```python
from build123d import *

# Parameters (mm, degrees)
SKETCH1_W           = 82
SKETCH1_H           = 82
BOSS_EXTRUDE1_DEPTH = 2
SKETCH2_R           = 7.955
CUT_EXTRUDE1_DEPTH  = 10
CUT_EXTRUDE4_DEPTH  = 10


with BuildPart() as part:
    # Sketch1 → Boss-Extrude1 (new body)
    with BuildSketch(Plane(origin=(0, 0, 0), x_dir=(1, 0, 0), z_dir=(0, 1, 0))):
        Rectangle(SKETCH1_W, SKETCH1_H)
    extrude(amount=BOSS_EXTRUDE1_DEPTH)

    # Sketch2 → Cut-Extrude1 (cut)
    with BuildSketch(Plane(origin=(0, 2, 0), x_dir=(1, 0, 0), z_dir=(0, 1, 0))):
        with Locations(Location((-12.87, 0, 0), (0, 0, 270))):
            Circle(SKETCH2_R)
        with Locations(Location((12.87, 0, 0), (0, 0, 270))):
            Circle(SKETCH2_R)
    extrude(amount=-CUT_EXTRUDE1_DEPTH, mode=Mode.SUBTRACT)

    # Sketch6 → Cut-Extrude4 (cut)
    with BuildSketch(Plane(origin=(0, 2, 0), x_dir=(1, 0, 0), z_dir=(0, 1, 0))):
        Polygon((-1.5, 22.5), (1.5, 22.5), (1.5, 28.3), (4, 28.3), (4, 31.75), (1.5, 31.75), (1.5, 41), (-1.5, 41), (-1.5, 31.75), (-4, 31.75), (-4, 28.3), (-1.5, 28.3), align=None)
        Polygon((28.3, 1.5), (28.3, 4), (31.75, 4), (31.75, 1.5), (41, 1.5), (41, -1.5), (31.75, -1.5), (31.75, -4), (28.3, -4), (28.3, -1.5), (22.5, -1.5), (22.5, 1.5), align=None)
        Polygon((1.5, -28.3), (4, -28.3), (4, -31.75), (1.5, -31.75), (1.5, -41), (-1.5, -41), (-1.5, -31.75), (-4, -31.75), (-4, -28.3), (-1.5, -28.3), (-1.5, -22.5), (1.5, -22.5), align=None)
        Polygon((-28.3, -1.5), (-28.3, -4), (-31.75, -4), (-31.75, -1.5), (-41, -1.5), (-41, 1.5), (-31.75, 1.5), (-31.75, 4), (-28.3, 4), (-28.3, 1.5), (-22.5, 1.5), (-22.5, -1.5), align=None)
    extrude(amount=-CUT_EXTRUDE4_DEPTH, mode=Mode.SUBTRACT)


solid = part.part
```
Part model, mm, in its own coordinate system. A direction names the side the tool comes from. Give positions to 0.01 mm unless a question says otherwise; leave off trailing zeros. Order: outer loops, then holes, each group sorted by start corner. A loop starts at its lowest first (then second) coordinate and runs counter-clockwise, first axis right, second up. Notation, with made-up numbers: M 21.5,-27.75 L 59.5,-27.75 A26 ccw 59.5,8.25 Z; hole C 49.25,-11.75 d6. An arc over 180 degrees is marked long. Use a Markdown table: item, result. Add a question column.
(1) Probe line 1 along X through (y, z) = (1.45, 0) (3 decimals); line 2 along Z through (x, y) = (29, 1.5); line 3 along Z through (x, y) = (26, 0.9). List the from-to ranges inside material, lowest first. Write a range as [from, to].
(2) Mould opens along Z. For faces 1 (the face through (0, 1, 22.5)), 2 (the face through (-1.5, 1, -36)), 3 (the face through (-36, 1, 1.5)), 4 (the face through (4, 1, 30)) say: +Z half, -Z half, draft (parallel to the pull), parting line (faces both ways), or undercut.
(3) 3-axis set-ups, long thin cutter, end or side, ignore diameter. For faces 5 (the face through (-1.5, 1, 36)), 6 (the face through (-25, 1, 1.5)), 7 (the face through (-3, 1, -28.3)): which of +Z, -Z, +X, -X, +Y, -Y reach the whole face in a straight line?
(4) Drop a flat-ended pin along its axis: P1, Ø4, axis at x = 8.5, z = 2.5, coming from the +Y side. Give the stop position or say it passes through.
(5) Saw through at D-D, the plane x = 24. Give the cut face in (y, z).
(6) Saw through at C-C, the plane y = 1.3. Give the number of separate pieces and of enclosed holes in the cut face, and give its area (3 significant figures).
(7) Saw through at A-A, the plane x = 12.87. Give the cut face in (y, z) (3 decimals), and give its area (3 significant figures).
(8) Saw through at B-B, the plane z = 0. Give the cut face in (x, y) (3 decimals), and give its area (3 significant figures).
Answer key:
| question | item | result |
|---|---|---|
| 1 | line 1 | [-22.5, -20.825], [-4.915, 4.915], [20.825, 22.5] |
| 1 | line 2 | [-41, -4], [4, 41] |
| 1 | line 3 | [-41, -1.5], [1.5, 41] |
| 2 | face 1 | +Z half |
| 2 | face 2 | draft |
| 2 | face 3 | undercut |
| 2 | face 4 | undercut |
| 3 | face 5 | +Z, +Y, -Y |
| 3 | face 6 | -X, +Y, -Y |
| 3 | face 7 | +Y, -Y |
| 4 | P1 | through |
| 5 | outline | M 0,-41 L 2,-41 L 2,-1.5 L 0,-1.5 Z; M 0,1.5 L 2,1.5 L 2,41 L 0,41 Z |
| 6 | separate pieces | 1 |
| 6 | enclosed holes | 2 |
| 6 | area | 6,040 mm^2 |
| 7 | outline | M 0,-41 L 2,-41 L 2,-7.955 L 0,-7.955 Z; M 0,7.955 L 2,7.955 L 2,41 L 0,41 Z |
| 7 | area | 132 mm^2 |
| 8 | outline | M -22.5,0 L -20.825,0 L -20.825,2 L -22.5,2 Z; M -4.915,0 L 4.915,0 L 4.915,2 L -4.915,2 Z; M 20.825,0 L 22.5,0 L 22.5,2 L 20.825,2 Z |
| 8 | area | 26.4 mm^2 |
